Verification items for the finished model (mm, model axes). A direction names the side the tool comes from. Coordinates: 2 decimals unless noted, no trailing zeros. Order: outer loops, then holes, each group sorted by start corner. A loop starts at its lowest first (then second) coordinate and runs counter-clockwise, first axis right, second up. Notation, with made-up numbers: (88, -7) -> (125, -7) arc R17 cw to (125, 18) -> close; hole circle Ø10 at (-21, 83.25). An arc over 180 degrees is marked (long way). Write each question's results on one line, items separated by ' | '. Start each with the question number.
(1) Go/stop test with flat-tipped pins: pin 1 (12.5 mm diameter, centred on y = -113, z = 106.5, fed in from +X); pin 2 (10.5 mm diameter, centred on y = -107.24, z = 127.55, fed in from -X); pin 3 (4 mm diameter, centred on y = -71.5, z = 127.5, fed in from +X); pin 4 (2.5 mm diameter, centred on y = -88.5, z = 54, fed in from +X). Record where each tip stops, or that it passes through.
(2) Cross-section at C-C on y = -174.5. Enter the section's corners in (x, z), and give its area (3 significant figures).
(3) Thickness scan on probe 1 along Y at (x, z) = (-1, 82); probe 2 along Y at (x, z) = (9, 134.5); probe 3 along Y at (x, z) = (-6, 37). Record the ranges inside material, lowest first. Write a range as [from, to].
(4) Cross-section at A-A on x = 29.5. Enter the section's corners in (y, z).
(5) Cross-section at B-B on y = -116. Enter the section's corners in (x, z), and give its area (3 significant figures).
(6) Set-up check for faces 1 (the flat face through (-5.15, -39, 82)), 2 (the cylindrical face through (-1.1, -110.2, 130.2)), 3 (the flat face through (-6, -215.9, 75)), 4 (the flat face through (-0.15, -114, 82)): record each of +Z, -Z, +X, -X, +Y, -Y from which the full face is reachable in a straight line by a thin tool's end or side.
(7) Draft check along X on faces 5 (the flat face through (-0.15, -157, 82)), 6 (the flat face through (-2.15, -68.5, 125.8)), 7 (the flat face through (-5, 38.1, 75)). Enter one of: +X half, -X half, draft (parallel to the pull), parting line (faces both ways), or undercut.
```python
from build123d import *

# Parameters (mm, degrees)
BOSS_EXTRUDE1_DEPTH = 152.4
BOSS_EXTRUDE2_DEPTH = 12.7
SKETCH3_R           = 1.984375
CUT_EXTRUDE1_DEPTH  = 25
SKETCH4_R           = 3.96875
CUT_EXTRUDE2_DEPTH  = 2


with BuildPart() as part:
    # Sketch1 → Boss-Extrude1 (new body)
    with BuildSketch(Plane(origin=(0, 0, 0), x_dir=(0, 1, 0), z_dir=(0, 0, 1))):
        with BuildLine():
            Line((-93.406104195, 5.15), (-84.393895805, 5.15))
            ThreePointArc((-84.393895805, 5.15), (-83.845691366, 4.849244745), (-83.804795744, 4.22529813))
            Line((-83.804795744, 4.22529813), (-85.141267349, 1.359225522))
            ThreePointArc((-85.141267349, 1.359225522), (-85.087788459, 0.543295333), (-84.37090573, 0.15))
            Line((-84.37090573, 0.15), (-43.036246445, 0.15))
            ThreePointArc((-43.036246445, 0.15), (-42.300124852, 0.575), (-42.300124852, 1.425))
            Line((-42.300124852, 1.425), (-43.887838092, 4.175))
            ThreePointArc((-43.887838092, 4.175), (-43.887838092, 4.825), (-43.324921579, 5.15))
            Line((-43.324921579, 5.15), (-34.393895805, 5.15))
            ThreePointArc((-34.393895805, 5.15), (-33.830979293, 4.825), (-33.830979293, 4.175))
            Line((-33.830979293, 4.175), (-35.418692533, 1.425))
            ThreePointArc((-35.418692533, 1.425), (-35.418692533, 0.575), (-34.68257094, 0.15))
            Line((-34.68257094, 0.15), (-7.5, 0.15))
            ThreePointArc((-7.5, 0.15), (-2.090633124, -2.090633124), (0.15, -7.5))
            Line((0.15, -7.5), (0.15, -12.5))
            ThreePointArc((0.15, -12.5), (-2.090633124, -17.909366876), (-7.5, -20.15))
            Line((-7.5, -20.15), (-24.85, -20.15))
            Line((-24.85, -20.15), (-24.85, -20))
            Line((-24.85, -20), (-25, -20))
            Line((-25, -20), (-25, -32.7))
            Line((-25, -32.7), (13.1, -32.7))
            ThreePointArc((13.1, -32.7), (30.77766953, -25.37766953), (38.1, -7.7))
            Line((38.1, -7.7), (38.1, 19.05))
            Line((38.1, 19.05), (-215.9, 19.05))
            Line((-215.9, 19.05), (-215.9, -7.7))
            ThreePointArc((-215.9, -7.7), (-208.57766953, -25.37766953), (-190.9, -32.7))
            Line((-190.9, -32.7), (-152.8, -32.7))
            Line((-152.8, -32.7), (-152.8, -20))
            Line((-152.8, -20), (-152.95, -20))
            Line((-152.95, -20), (-152.95, -20.15))
            Line((-152.95, -20.15), (-170.3, -20.15))
            ThreePointArc((-170.3, -20.15), (-175.709366876, -17.909366876), (-177.95, -12.5))
            Line((-177.95, -12.5), (-177.95, -7.5))
            ThreePointArc((-177.95, -7.5), (-175.709366876, -2.090633124), (-170.3, 0.15))
            Line((-170.3, 0.15), (-143.036246445, 0.15))
            ThreePointArc((-143.036246445, 0.15), (-142.300124852, 0.575), (-142.300124852, 1.425))
            Line((-142.300124852, 1.425), (-143.887838092, 4.175))
            ThreePointArc((-143.887838092, 4.175), (-143.887838092, 4.825), (-143.324921579, 5.15))
            Line((-143.324921579, 5.15), (-134.393895805, 5.15))
            ThreePointArc((-134.393895805, 5.15), (-133.830979293, 4.825), (-133.830979293, 4.175))
            Line((-133.830979293, 4.175), (-135.418692533, 1.425))
            ThreePointArc((-135.418692533, 1.425), (-135.418692533, 0.575), (-134.68257094, 0.15))
            Line((-134.68257094, 0.15), (-93.11742906, 0.15))
            ThreePointArc((-93.11742906, 0.15), (-92.381307467, 0.575), (-92.381307467, 1.425))
            Line((-92.381307467, 1.425), (-93.969020707, 4.175))
            ThreePointArc((-93.969020707, 4.175), (-93.969020707, 4.825), (-93.406104195, 5.15))
        make_face()
    extrude(amount=BOSS_EXTRUDE1_DEPTH)

    # Sketch2 → Boss-Extrude2 (add)
    with BuildSketch(Plane(origin=(0, 0, 0), x_dir=(1, 0, 0), z_dir=(0, 0, -1))):
        Polygon((-19.05, 215.9), (-19.05, -38.1), (7.7, -38.1), (32.7, 25), (32.7, 152.8), (32.7, 190.9), (7.7, 215.9), align=None)
    extrude(amount=-BOSS_EXTRUDE2_DEPTH)

    # Sketch3 → Cut-Extrude1 (cut)
    with BuildSketch(Plane.YZ.offset(-0.15)):
        with Locations((-107.244167395, 37.55)):
            Circle(SKETCH3_R)
        with Locations((-107.244167395, 82.55)):
            Circle(SKETCH3_R)
        with Locations((-107.244167395, 127.55)):
            Circle(SKETCH3_R)
        with Locations((-70.244167395, 37.55)):
            Circle(SKETCH3_R)
        with Locations((-70.244167395, 82.55)):
            Circle(SKETCH3_R)
        with Locations((-70.244167395, 127.55)):
            Circle(SKETCH3_R)
    extrude(amount=-CUT_EXTRUDE1_DEPTH, mode=Mode.SUBTRACT)

    # Sketch4 → Cut-Extrude2 (cut)
    with BuildSketch(Plane.YZ.offset(-0.15)):
        with Locations((-107.244167395, 127.55)):
            Circle(SKETCH4_R)
        with Locations((-107.244167395, 82.55)):
            Circle(SKETCH4_R)
        with Locations((-107.244167395, 37.55)):
            Circle(SKETCH4_R)
        with Locations((-70.244167395, 37.55)):
            Circle(SKETCH4_R)
        with Locations((-70.244167395, 82.55)):
            Circle(SKETCH4_R)
        with Locations((-70.244167395, 127.55)):
            Circle(SKETCH4_R)
    extrude(amount=-CUT_EXTRUDE2_DEPTH, mode=Mode.SUBTRACT)


solid = part.part
```
Results are:
1) pin 1: stops at x = -0.15 | pin 2: stops at x = -19.05 | pin 3: stops at x = -2.15 | pin 4: stops at x = -5.15
2) outline: (-19.05, 0) -> (32.7, 0) -> (32.7, 152.4) -> (18.89, 152.4) -> (18.89, 12.7) -> (1.11, 12.7) -> (1.11, 152.4) -> (-19.05, 152.4) -> close | area: 5,400 mm2
3) probe 1: y = [-215.9, -142.19], [-135.53, -111.17], [-103.31, -92.27], [-85.22, -74.17], [-66.31, -42.19], [-35.53, 38.1] | probe 2: y = [-215.87, -177.95], [0.15, 38.07] | probe 3: y = [-215.9, -109.15], [-105.34, -72.15], [-68.34, 38.1]
4) outline: (-203.14, 0) -> (25.34, 0) -> (25.34, 152.4) -> (-25, 152.4) -> (-25, 12.7) -> (-152.8, 12.7) -> (-152.8, 152.4) -> (-203.14, 152.4) -> close
5) outline: (-19.05, 0) -> (32.7, 0) -> (32.7, 12.7) -> (-0.15, 12.7) -> (-0.15, 152.4) -> (-19.05, 152.4) -> close | area: 3,300 mm2
6) face 1: +Z | face 2: +X | face 3: +Z, -Z, +X, -X, -Y | face 4: +Z, +X
7) face 5: undercut | face 6: +X half | face 7: draft
